Design review of the part built by this model. Coordinates are the model's own, in mm. Coordinates: 2 decimals unless noted, no trailing zeros. Loops run counter-clockwise (first coordinate to the right, second up) from the corner with the lowest first, then second, coordinate; pieces in that order, holes last. Notation, with made-up numbers: M -28.75,47 L -17.75,47 A22 cw -17.75,64 Z; hole C 84,66 d8. An arc over 180 degrees is marked long. Put each result on its own line as item: value. Start each with the question number.
(1) Take a section at A-A, the plane x = 109.5. Give the boundary of the cut face in (y, z) (3 decimals), then the cut area to 3 significant figures.
(2) Clearance check with flat-ended pins moving along their axes: pin 1 (1.5 mm diameter, centred on x = 155.5, y = -3, fed in from +Z); pin 2 (1 mm diameter, centred on x = 76, y = -1.5, fed in from -Z). State where each tip first meets the part, or that it passes through.
(3) For probe 1 along Z at (x, y) = (46, -1.8); probe 2 along X at (y, z) = (-0.05, 18); probe 3 along Z at (x, y) = (156.5, -1.3), list the stretches that pass through material, from the lowest coordinate up. Write a range as [from, to].
```python
from build123d import *

# Parameters (mm, degrees)
F1_DEPTH = 3.175


with BuildPart() as f1:
    # F0 (on Front) → F1 (new body)
    with BuildSketch(Plane.XZ):
        with BuildLine():
            Line((122.3122592662, 33.7521504266), (-55.4877407338, 33.7521504266))
            Line((-55.4877407338, 33.7521504266), (-55.3766458406, 28.9909463589))
            Line((-55.3766458406, 28.9909463589), (122.3122592662, 28.9909463589))
            add(Edge.make_bspline(
                [(185.8122592662, -9.1090536411), (185.8122592662, 28.9909463589), (122.3122592662, 28.9909463589)],
                knots=[0, 0, 0, 1.5707963268, 1.5707963268, 1.5707963268], degree=2, weights=[1, 0.7071067812, 1]))
            Line((185.8122592662, -9.1090536411), (190.5747592662, -9.1090536411))
            add(Edge.make_bspline(
                [(190.5747592662, -9.1090536411), (190.5747592662, 33.7534463589), (122.3122592662, 33.7534463589)],
                knots=[0, 0, 0, 1.5707963268, 1.5707963268, 1.5707963268], degree=2, weights=[1, 0.7071067812, 1]))
            Line((122.3122592662, 33.7534463589), (122.3122592662, 33.7521504266))
        make_face()
    extrude(amount=F1_DEPTH)


solid = f1.part
```
Computed values:
1. outline: M -3.175,28.991 L 0,28.991 L 0,33.752 L -3.175,33.752 Z
1. area: 15.1 mm^2
2. pin 1: stops at z = 28.6
2. pin 2: stops at z = 28.99
3. probe 1: z = [28.99, 33.75]
3. probe 2: x = [166.93, 175.19]
3. probe 3: z = [23, 27.99]
